Model file for the job. Use its own axes, mm. A direction names the side the tool comes from. Give positions to 0.01 mm unless a question says otherwise; leave off trailing zeros. Loops run counter-clockwise (first coordinate to the right, second up) from the corner with the lowest first, then second, coordinate; pieces in that order, holes last. Notation, with made-up numbers: (76, 75) -> (132, 75) arc R18 ccw to (132, 102) -> close; hole circle Ø9 at (66, 57). An arc over 180 degrees is marked (long way). Use CSV: the item, a comma, the result in double quotes. Start each with the question number.
(1) 3-axis set-ups, long thin cutter, end or side, ignore diameter. For faces 4 (the flat face through (-8, -10, 0)), 5 (the flat face through (-10, -5, 0)): which of +Z, -Z, +X, -X, +Y, -Y reach the whole face in a straight line?
(2) Drill centre lines: probe 1 along Z at (x, y) = (0, -10.5); probe 2 along Y at (x, z) = (-8.25, 8.25); probe 3 along X at (y, z) = (-9.25, 0). Where is each one in solid material? Low to high.
(3) Pull direction X, two halves, no side cores. Call faces 1 (the cylindrical face through (9.699, -0.285, 0.126)), 2 (the cylindrical face through (-9.715, -9.699, 0.633)), 3 (the cylindrical face through (-5, -10.9, 1.6)): pulls with the +X half, pulls with the -X half, needs draft (parallel to the pull), parting line crosses it, or undercut.
(4) Cut at A-A on x = -8. Write the cut outline in (y, z).
from build123d import *

# Parameters (mm, degrees)
F0_W     = 20
F0_H     = 20
F1_DEPTH = 10
F2_R     = 7.5
F3_DEPTH = 5
F5_D     = 10.5
F5_DEPTH = 8
F5_TIP   = 3.1545182499
F6_R     = 1
F7_SIZE  = 0.5


with BuildPart() as f1:
    # F0 (on Front) → F1 (new body)
    with BuildSketch(Plane.XZ):
        Rectangle(F0_W, F0_H)
    extrude(amount=F1_DEPTH)

    # F2 (on face) → F3 (join)
    with BuildSketch(Plane.XZ.offset(10)):
        Circle(F2_R)
    extrude(amount=F3_DEPTH)

    # F5
    with Locations(Plane.XZ.offset(15)):
        with Locations((0, 0)):
            Hole(F5_D / 2, depth=F5_DEPTH)
            with Locations((0, 0, -(F5_DEPTH + F5_TIP / 2))):  # 118° drill point
                Cone(0, F5_D / 2, F5_TIP, mode=Mode.SUBTRACT)

    # F6
    f6_edges = [f1.edges().sort_by_distance(p)[0] for p in [
        (0, -10, 10),
        (-10, -10, 0),
        (0, -10, -10),
        (10, -10, 0),
        (-10, -5, -10),
        (0, 0, -10),
        (10, -5, -10),
        (10, -5, 10),
        (10, 0, 0),
        (-10, 0, 0),
        (0, 0, 10),
    ]]
    fillet(f6_edges, radius=F6_R)

    # F7
    f7_edges = [f1.edges().sort_by_distance(p)[0] for p in [
        (-7.5, -15, 0),
    ]]
    chamfer(f7_edges, length=F7_SIZE)


solid = f1.part
Check result:
1,face 4,"-Y"
1,face 5,"+Z, -Z, -X, +Y, -Y"
2,probe 1,"-7.5 to -5.25, 5.25 to 7.5"
2,probe 2,"-10 to 0"
2,probe 3,"-9.97 to -5.25, 5.25 to 9.97"
3,face 1,"pulls with the +X half"
3,face 2,"pulls with the -X half"
3,face 3,"undercut"
4,outline,"(-10, -9) arc R1 ccw to (-9, -10) -> (-1, -10) arc R1 ccw to (0, -9) -> (0, 9) arc R1 ccw to (-1, 10) -> (-9, 10) arc R1 ccw to (-10, 9) -> close"
